Autodesk Inventor part; units mm, degrees
ref_plane "作業平面1" through (0, 0, 0.5) normal (0, 0, 1) x (1, 0, 0)
ref_plane "作業平面3" through (-10.25, -17.7535, -28.7) normal (-0.5, -0.866, 0) x (0, 0, -1)
ref_plane "YZ Plane" through (0, 0, 0) normal (1, 0, 0) x (0, 1, 0)
sketch "スケッチ1" plane through (0, 0, 0) normal (0, 0, 1) x (1, 0, 0)
  circle A0 centre (0, 0) radius 15
  dimension "d0" = 30
extrude "押し出し1" add sketch "スケッチ1" against normal blind 11.5
sketch "スケッチ2" plane through (0, 0, 0) normal (0, 0, 1) x (1, 0, 0)
  circle A0 centre (0, 6.5) radius 3
  point P0 (0, 0)
  dimension "d3" = 6
  dimension "d4" = 6.5
extrude "押し出し2" add sketch "スケッチ2" along normal blind 1.5
sketch "スケッチ3" plane through (0, 6.5, 1.5) normal (0, 0, 1) x (1, 0, 0)
  circle A0 centre (0, 0) radius 3
  circle A1 centre (0, 0) radius 1.5
  point P0 (0, -6.5)
  dimension "d7" = 3
extrude "押し出し3" add sketch "スケッチ3" along normal blind 10 contours A1
sketch "スケッチ4" plane through (0, 0, -11.5) normal (0, 0, -1) x (-1, 0, 0)
  circle A0 centre (0, 0) radius 13.5
  dimension "d10" = 27
extrude "押し出し4" add sketch "スケッチ4" along normal blind 17.2
sketch "スケッチ6" plane through (0, 6.5, 11.5) normal (0, 0, 1) x (1, 0, 0)
  circle A0 centre (0, 0) radius 1.5
  line L0 (-1.118, 1) -> (1.118, 1)
  point P0 (0, -6.5)
  dimension "d21" = 1
extrude "押し出し6" cut sketch "スケッチ6" against normal blind 8 contours L0 A0 picked at (-0.0599, 1.1631)
ref_plane "作業平面1" through (0, 0, 0.5) normal (0, 0, 1) x (1, 0, 0)
sketch "スケッチ7" plane through (0, 0, 0.5) normal (0, 0, 1) x (1, 0, 0)
  line L0 (0, 21.4774) -> (0, -21.4774) construction
  line L1 (-14.5, 6) -> (-13.5, 6)
  line L2 (-13.5, 6) -> (-13.5, -6)
  line L3 (-13.5, -6) -> (-14.5, -6)
  line L4 (-14.5, -6) -> (-14.5, 6)
  line L5 (13.5, 6) -> (14.5, 6)
  line L6 (14.5, 6) -> (14.5, -6)
  line L7 (14.5, -6) -> (13.5, -6)
  line L8 (13.5, -6) -> (13.5, 6)
  circle A0 centre (-18.5, 0) radius 1.75
  circle A1 centre (18.5, 0) radius 1.75
  circle A2 centre (-18.5, 0) radius 3.5
  circle A3 centre (18.5, 0) radius 3.5
  line L9 (-14.5, 6) -> (-20.1038, 3.1109)
  line L10 (-20.1038, -3.1109) -> (-14.5, -6)
  line L11 (14.5, 6) -> (20.1038, 3.1109)
  line L12 (20.1038, -3.1109) -> (14.5, -6)
  point P0 (0, 0)
  point P1 (0, 0)
  point P2 (-13.5, 0)
  point P3 (13.5, 0)
  dimension "d25" = 1
  dimension "d26" = 12
  dimension "d27" = 29
  dimension "d28" = 3.5
  dimension "d29" = 37
  dimension "d30" = 7
extrude "押し出し7" add sketch "スケッチ7" against normal blind 1
ref_plane "作業平面3" through (-10.25, -17.7535, -28.7) normal (-0.5, -0.866, 0) x (0, 0, -1)
ref_plane "作業平面2" through (0, 0, -28.7) normal (-0.5, -0.866, 0) x (0, 0, -1)
sketch "スケッチ9" plane through (-10.25, -17.7535, -28.7) normal (-0.5, -0.866, 0) x (0, 0, -1)
  line L0 (-11.8, -5.25) -> (-8.1, -5.25)
  line L1 (-8.1, -5.25) -> (-8.1, 5.25)
  line L2 (-8.1, 5.25) -> (-11.8, 5.25)
  line L3 (-11.8, 5.25) -> (-11.8, -5.25)
  line L4 (-29.2, -15.855) -> (-29.2, -9.5574)
  point P0 (-28.7, 0)
  point P1 (-11.8, 0)
  dimension "d35" = 3.7
  dimension "d36" = 10.5
  dimension "d37" = 17.4
extrude "押し出し8" add sketch "スケッチ9" against normal blind 4
sketch "スケッチ10" plane through (-8.25, -14.2894, -28.7) normal (0.5, 0.866, 0) x (0.866, -0.5, 0)
  line L0 (-6, -4.9) -> (6, -4.9)
  line L1 (6, -4.9) -> (6, -14.3)
  line L2 (6, -14.3) -> (-6, -14.3)
  line L3 (-6, -14.3) -> (-6, -4.9)
  line L4 (-15.855, -29.2) -> (-9.5574, -29.2)
  point P0 (0, -28.7)
  point P1 (0, -14.3)
  dimension "d40" = 12
  dimension "d41" = 9.4
  dimension "d42" = 14.9
extrude "押し出し9" add sketch "スケッチ10" along normal blind 4
properties part number "SPG27"
Could you check a few things on this model? Use its own coordinates, in mm. A direction names the side the tool comes from. Give positions to 0.01 mm unless a question says otherwise; leave off trailing zeros. Order: outer loops, then holes, each group sorted by start corner. A loop starts at its lowest first (then second) coordinate and runs counter-clockwise, first axis right, second up. Notation, with made-up numbers: (-27, 77) - (4, 77) arc R35 cw to (4, 115) - close; hole circle Ø11 at (10.25, -40). An arc over 180 degrees is marked (long way). Return JSON: item names as keys, results as strings. Group by question number.
Q1. Suppose I cut it at B-B, the plane x = 18.5. Please give me the cut outline in (y, z).
Q2. Will these pins go through, and if not, where does the flat tip stop? pin 1 Ø6.5 at (x, y) = (-17, -2.5) entering from -Z; pin 2 Ø8 at (y, z) = (4.5, -18.5) entering from +X; pin 3 Ø1.5 at (x, y) = (-11.5, -2.5) entering from +Z; pin 4 Ø13.5 at (x, y) = (3.5, 6.5) entering from +Z.
Q3. Suppose I cut it at D-D, the plane y = -16. Please give me the cut outline in (x, z), and give its area (3 significant figures).
Q4. Which directions (+Z, -Z, +X, -X, +Y, -Y) give clear straight access to the entire face, cutting with the end or side of a thin tool? Please do faces 4 (the face through (-16, 0, 0.5)), 5 (the face through (-13.8, -13.4, -18.7)), 6 (the face through (16, 0, 0.5)), 7 (the face through (0, 5, 6)), 8 (the face through (-9, -16, -20.6)).
Q5. Please list where these lines run through material, in increasing order: line 1 along Z through (x, y) = (-7, -13); line 2 along Y through (x, z) = (-18.5, 0.15); line 3 along Z through (x, y) = (6.5, -3). Write a range as [from, to].
Q6. Suppose I cut it at C-C, the plane z = -22. Please give me the cut outline in (x, y).
Q7. Thinking about a two-plate mould opening in Y: for faces 1 (the face through (-20.25, 0.08, 0.01)), 2 (the face through (-9, -16, -16.9)), 3 (the face through (-14.985, 0.66, -5.67)), which applies, pulls with the +Y half, pulls with the -Y half, needs draft (parallel to the pull), parting line crosses it, or undercut?
Q8. Suppose I cut it at A-A, the plane y = 0. Please give me the cut outline in (x, z), and give its area (3 significant figures).
Resolved:
{
 "1": {"outline": "(-3.94, -0.5) - (-1.75, -0.5) - (-1.75, 0.5) - (-3.94, 0.5) - close; (1.75, -0.5) - (3.94, -0.5) - (3.94, 0.5) - (1.75, 0.5) - close"},
 "2": {"pin 1": "stops at z = -11.5", "pin 2": "stops at x = 13.49", "pin 3": "stops at z = 0", "pin 4": "stops at z = 11.5"},
 "3": {"outline": "(-13.29, -20.6) - (-5.29, -20.6) - (-5.29, -23.8) - (-2.31, -23.8) - (-2.31, -14.4) - (-5.29, -14.4) - (-5.29, -16.9) - (-13.29, -16.9) - close", "area": "57.6 mm2"},
 "4": {"face 4": "+Z, -X, +Y, -Y", "face 5": "+Z, -Z, -X", "face 6": "+Z, +X, +Y, -Y", "face 7": "+Z", "face 8": "-Z, -X, -Y"},
 "5": {"line 1": "z = [-23.8, -14.4], [-11.5, 0]", "line 2": "y = [-3.94, -1.75], [1.75, 3.94]", "line 3": "z = [-28.7, 0]"},
 "6": {"outline": "(-13.45, -11.29) - (-3.05, -17.29) - (-1.05, -13.83) - (-1.83, -13.37) arc R13.5 ccw (long way) to (-10.67, -8.28) - (-11.45, -7.83) - close"},
 "7": {"face 1": "undercut", "face 2": "needs draft", "face 3": "parting line crosses it"},
 "8": {"outline": "(-22, -0.5) - (-20.25, -0.5) - (-20.25, 0.5) - (-22, 0.5) - close; (-16.75, -0.5) - (-15, -0.5) - (-15, -11.5) - (-13.5, -11.5) - (-13.5, -28.7) - (13.5, -28.7) - (13.5, -11.5) - (15, -11.5) - (15, -0.5) - (16.75, -0.5) - (16.75, 0.5) - (13.5, 0.5) - (13.5, 0) - (-13.5, 0) - (-13.5, 0.5) - (-16.75, 0.5) - close; (20.25, -0.5) - (22, -0.5) - (22, 0.5) - (20.25, 0.5) - close", "area": "818 mm2"}
}
